Drawing for the job (mm, zero at the part's lowest x, y, z). Give positions to 0.01 mm unless a question says otherwise; leave off trailing zeros. Loops run counter-clockwise (first coordinate to the right, second up) from the corner with the lowest first, then second, coordinate; pieces in that order, holes last. Notation, with made-up numbers: (55, -5.5) -> (101, -5.5) arc R8 ccw to (101, 6.5) -> close; hole circle Ø7 at (-14, -18.75). An arc over 180 degrees is marked (long way). Use CSV: the item, a comma, the result in double quotes. Start each with the question number.
(1) Drill centre lines: probe 1 along X at (y, z) = (14, 37.5); probe 2 along Z at (x, y) = (38, 32); probe 3 along Z at (x, y) = (55.5, 27.5). Where is each one in solid material? Low to high.
(2) Pull direction Z, two halves, no side cores. Call the marked faces 1, 2, 3 and 4: pulls with the +Z half, pulls with the -Z half, needs draft (parallel to the pull), parting line crosses it, or undercut.
(3) Cut at D-D on y = 3. Write the cut outline in (x, z).
(4) Cut at C-C on y = 28. Write the cut outline in (x, z), then the cut area to 3 significant figures.
(5) Cut at A-A on x = 38.1. Write the cut outline in (y, z).
(6) Flat gauge pin, fed straight in: pin 1 (8 mm diameter, centred on x = 68.5, y = 12.5, fed in from -Z). Where does the tip first touch, or does it go through?
(7) Cut at B-B on z = 38.1. Write the cut outline in (x, y), then the cut area to 3 significant figures.
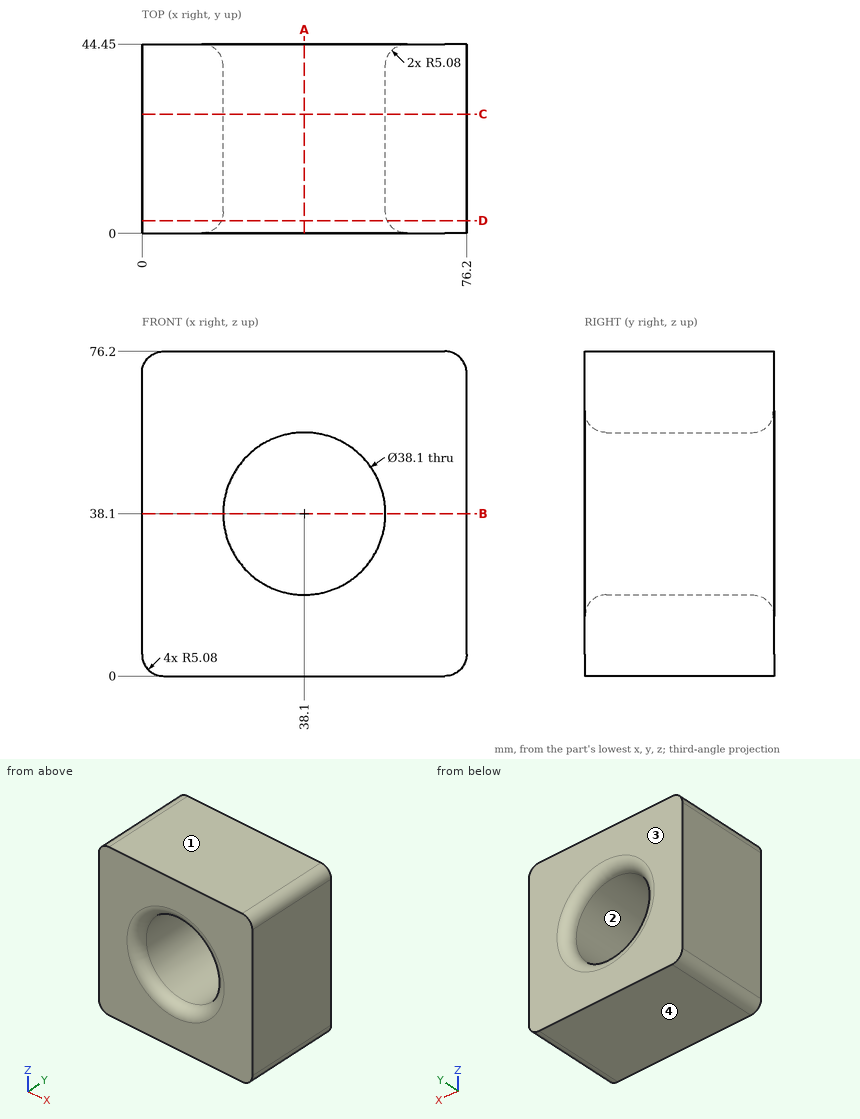
Check result:
1,probe 1,"0 to 19.06, 57.14 to 76.2"
1,probe 2,"0 to 19.05, 57.15 to 76.2"
1,probe 3,"0 to 30.34, 45.86 to 76.2"
2,face 1,"pulls with the +Z half"
2,face 2,"undercut"
2,face 3,"needs draft"
2,face 4,"pulls with the -Z half"
3,outline,"(0, 5.08) arc R5.08 ccw to (5.08, 0) -> (71.12, 0) arc R5.08 ccw to (76.2, 5.08) -> (76.2, 71.12) arc R5.08 ccw to (71.12, 76.2) -> (5.08, 76.2) arc R5.08 ccw to (0, 71.12) -> close; hole circle Ø38.99 at (38.1, 38.1)"
4,outline,"(0, 5.08) arc R5.08 ccw to (5.08, 0) -> (71.12, 0) arc R5.08 ccw to (76.2, 5.08) -> (76.2, 71.12) arc R5.08 ccw to (71.12, 76.2) -> (5.08, 76.2) arc R5.08 ccw to (0, 71.12) -> close; hole circle Ø38.1 at (38.1, 38.1)"
4,area,"4,640 mm²"
5,outline,"(0, 0) -> (44.45, 0) -> (44.45, 13.97) arc R5.08 ccw to (39.37, 19.05) -> (5.08, 19.05) arc R5.08 ccw to (0, 13.97) -> close; (0, 62.23) arc R5.08 ccw to (5.08, 57.15) -> (39.37, 57.15) arc R5.08 ccw to (44.45, 62.23) -> (44.45, 76.2) -> (0, 76.2) -> close"
6,pin 1,"z = 0"
7,outline,"(0, 0) -> (13.97, 0) arc R5.08 ccw to (19.05, 5.08) -> (19.05, 39.37) arc R5.08 ccw to (13.97, 44.45) -> (0, 44.45) -> close; (57.15, 5.08) arc R5.08 ccw to (62.23, 0) -> (76.2, 0) -> (76.2, 44.45) -> (62.23, 44.45) arc R5.08 ccw to (57.15, 39.37) -> close"
7,area,"1,670 mm²"
